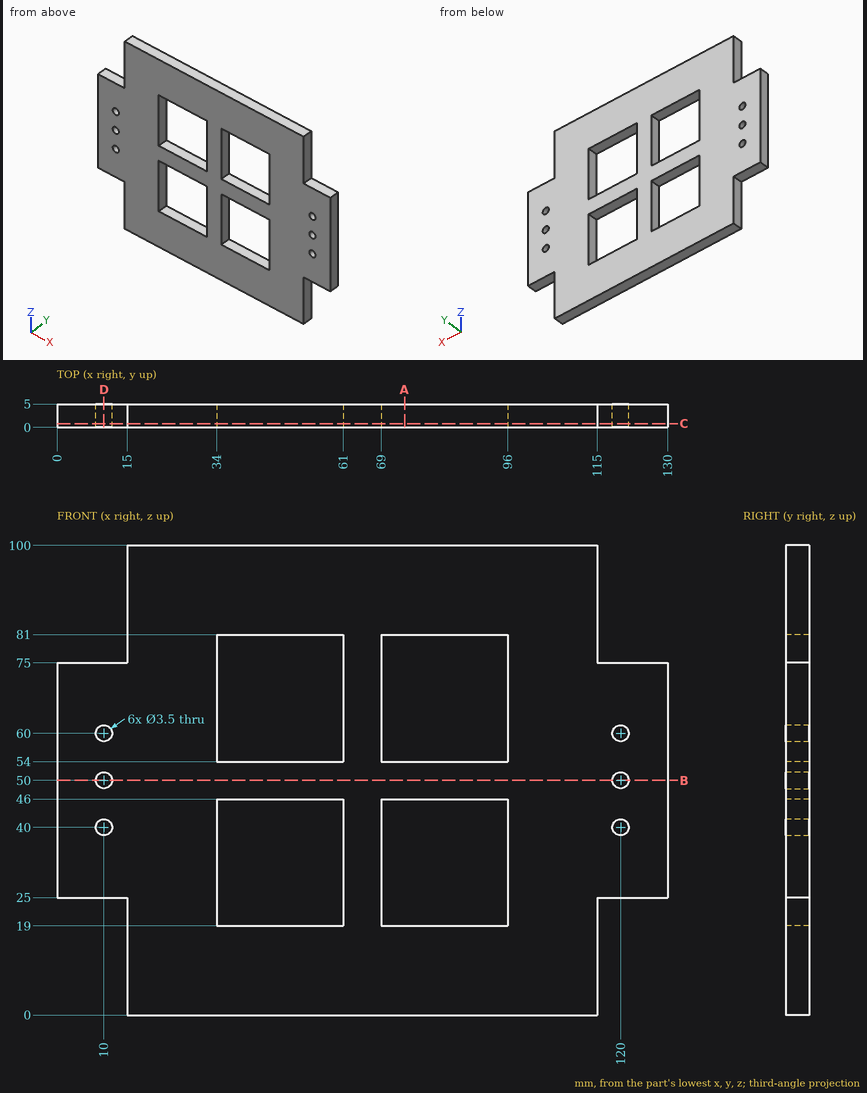
The figure shows three views and two pictorial views of one solid part (mm, origin at its lowest corner). Answer the questions. Give positions to 0.01 mm unless a question says otherwise; leave off trailing zeros. Write each loop counter-clockwise with the first axis right and the second up, starting at its lowest first coordinate (ties: lowest second). Pieces come first, ordered by that corner, then holes. Notation, with made-up numbers: M 48,20.25 L 94,20.25 A30 ccw 94,58.25 Z; hole C -19,-35 d3. An arc over 180 degrees is marked long. One line per item, written item: value. Start each with the question number.
(1) Find section A-A (x = 74). Determine the outline of the cut face in (y, z).
(2) Find section D-D (x = 10). Determine the outline of the cut face in (y, z).
(3) Find section C-C (y = 0.8). Give the number of separate pieces and of enclosed holes in the cut face, plus the area to 3 significant figures.
(4) Find the intervals of material crossed by line 1 (Z direction, x = 51, y = 3.6); line 2 (X direction, y = 3.7, z = 50); line 3 (X direction, y = 0.55, z = 32.5), in increasing order.
(5) Find section B-B (z = 50). Determine the outline of the cut face in (x, y), plus the area to 3 significant figures.
Results below:
1. outline: M 0,0 L 5,0 L 5,19 L 0,19 Z; M 0,46 L 5,46 L 5,54 L 0,54 Z; M 0,81 L 5,81 L 5,100 L 0,100 Z
2. outline: M 0,25 L 5,25 L 5,38.25 L 0,38.25 Z; M 0,41.75 L 5,41.75 L 5,48.25 L 0,48.25 Z; M 0,51.75 L 5,51.75 L 5,58.25 L 0,58.25 Z; M 0,61.75 L 5,61.75 L 5,75 L 0,75 Z
3. separate pieces: 1
3. enclosed holes: 10
3. area: 8,530 mm^2
4. line 1: z = 0 to 19, 46 to 54, 81 to 100
4. line 2: x = 0 to 8.25, 11.75 to 118.25, 121.75 to 130
4. line 3: x = 0 to 34, 61 to 69, 96 to 130
5. outline: M 0,0 L 8.25,0 L 8.25,5 L 0,5 Z; M 11.75,0 L 118.25,0 L 118.25,5 L 11.75,5 Z; M 121.75,0 L 130,0 L 130,5 L 121.75,5 Z
5. area: 615 mm^2
